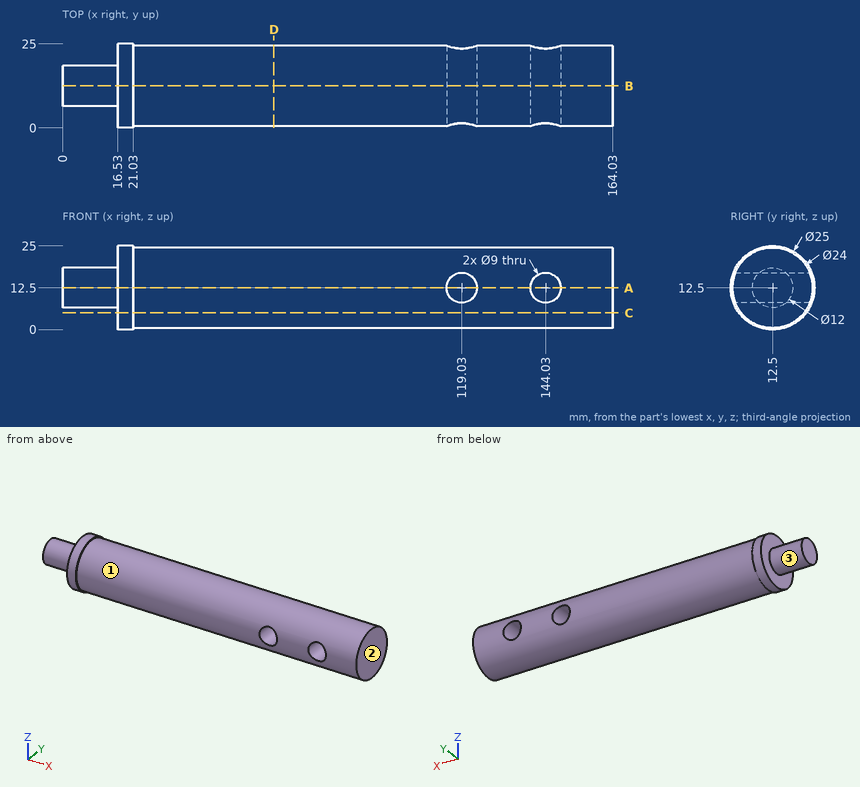
The figure shows three views and two pictorial views of one solid part (mm, origin at its lowest corner). Answer the questions. A direction names the side the tool comes from. Give positions to 0.01 mm unless a question says otherwise; leave off trailing zeros. Order: outer loops, then holes, each group sorted by start corner. A loop starts at its lowest first (then second) coordinate and runs counter-clockwise, first axis right, second up. Notation, with made-up numbers: M 20.5,88 L 37.5,88 A35 ccw 37.5,123 Z; hole C 88,47.25 d2. An arc over 180 degrees is marked long. Return JSON: item names as keys, results as strings.
Q1. Find section B-B, the plane y = 12.5. Write down the section's boundary in (x, z), and give its area (3 significant figures).
Answer below:
{"outline": "M 0,6.5 L 16.53,6.5 L 16.53,0 L 21.03,0 L 21.03,0.5 L 164.03,0.5 L 164.03,24.5 L 21.03,24.5 L 21.03,25 L 16.53,25 L 16.53,18.5 L 0,18.5 Z; hole C 119.03,12.5 d9; hole C 144.03,12.5 d9", "area": "3,620 mm^2"}
Q2. Which of the six approach directions +Z, -Z, +X, -X, +Y, -Y give full straight-line access (tool end or side, diameter ignored) to the marked faces 1, 2 and 3?
Answer below:
{"face 1": "+X", "face 2": "+Z, -Z, +X, +Y, -Y", "face 3": "-X"}
Q3. Find section A-A, the plane z = 12.5. Write down the section's boundary in (x, y), and give its area (3 significant figures).
Answer below:
{"outline": "M 0,6.5 L 16.53,6.5 L 16.53,0 L 21.03,0 L 21.03,0.5 L 114.53,0.5 L 114.53,24.5 L 21.03,24.5 L 21.03,25 L 16.53,25 L 16.53,18.5 L 0,18.5 Z; M 123.53,0.5 L 139.53,0.5 L 139.53,24.5 L 123.53,24.5 Z; M 148.53,0.5 L 164.03,0.5 L 164.03,24.5 L 148.53,24.5 Z", "area": "3,310 mm^2"}
Q4. Each of these flat-tipped pins is pushed along its axis until it touches: pin 1 (8 mm diameter, centred on x = 82, z = 14, fed in from +Y); pin 2 (10 mm diameter, centred on x = 131, y = 11, fed in from -Z); pin 3 (3 mm diameter, centred on y = 4.5, z = 21, fed in from -X). Where does it stop, or does it pass through?
Answer below:
{"pin 1": "stops at y = 24.5", "pin 2": "stops at z = 0.5", "pin 3": "stops at x = 16.53"}
Q5. Find section D-D, the plane x = 63. Write down the section's boundary in (y, z).
Answer below:
{"outline": "C 12.5,12.5 d24"}
Q6. Find the intervals of material crossed by line 1 along X through (y, z) = (8.5, 12.5); line 2 along Z through (x, y) = (144.03, 12.75); line 3 along X through (y, z) = (14, 11.75), in increasing order. Write a range as [from, to].
Answer below:
{"line 1": "x = [0, 114.53], [123.53, 139.53], [148.53, 164.03]", "line 2": "z = [0.5, 8], [17, 24.5]", "line 3": "x = [0, 114.59], [123.47, 139.59], [148.47, 164.03]"}
Q7. Find section C-C, the plane z = 5. Write down the section's boundary in (x, y), and give its area (3 significant figures).
Answer below:
{"outline": "M 16.53,2.5 L 21.03,2.5 L 21.03,3.13 L 164.03,3.13 L 164.03,21.87 L 21.03,21.87 L 21.03,22.5 L 16.53,22.5 Z", "area": "2,770 mm^2"}
